Geometry: final body of the model. Coordinates: model frame, mm. Face numbers are marked on the shaded views. A direction names the side the tool comes from. Give positions to 0.01 mm unless a question says otherwise; leave off trailing zeros. Write each loop counter-clockwise with the first axis right and the second up, starting at its lowest first coordinate (ties: lowest second). Pieces come first, ordered by that corner, then holes.
Q1. Section D-D (y = 5.5). Return the cut outline in (x, z), plus the area to 3 significant figures.
Q2. Section B-B (x = 5). Return the cut outline in (y, z).
Q3. Reachability of the marked faces 4, 5 and 6 from +Z, -Z, +X, -X, +Y, -Y: full face, straight path, thin tool, end or side. Return the list, or none.
Q4. Pin query (flat end, axial travel): pin 1 Ø0.5 at (x, y) = (57.5, 1.5) entering from -Z; pin 2 Ø6 at (x, z) = (33.5, -56) entering from +Y; pin 3 Ø1 at (x, y) = (7.5, 2) entering from -Z. Return the tip coordinate at first contact, or that it passes through.
Q5. Line query: line 1 (Z direction, x = 24, y = 12.5); line 2 (X direction, y = 15, z = -29); line 3 (Z direction, x = 32, y = 11). Output: solid intervals per line, ascending.
Q6. Mould query, pull axis X, two halves, no side actions, for the marked faces 1, 2 and 3. Classes: +X half, -X half, draft (parallel to the pull), parting line (faces both ways), or undercut.
Q7. Section A-A (y = 12.25). Return the cut outline in (x, z).
Q8. Section C-C (z = -53.5). Return the cut outline in (x, y).
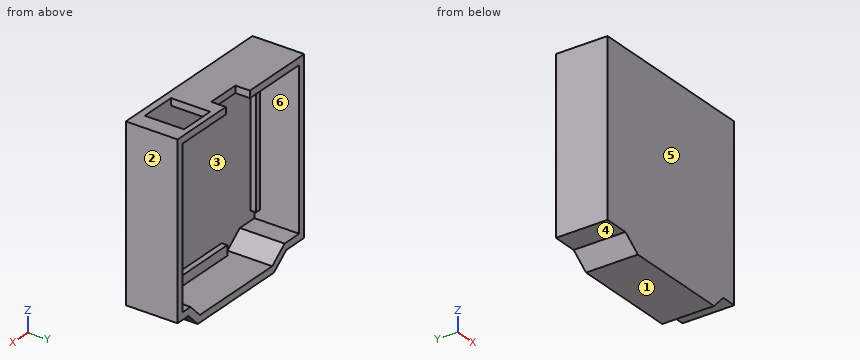
from build123d import *

# Parameters (mm, degrees)
BOSS_EXTRUDE1_DEPTH = 16
SHELL1_T            = 2.5
SKETCH2_W           = 13
SKETCH2_H           = 14
SKETCH2_W_2         = 12
SKETCH2_H_2         = 5.195244662
CUT_EXTRUDE1_DEPTH  = 4
SKETCH3_W           = 2
SKETCH3_H           = 50
SKETCH3_W_2         = 1.814522713
BOSS_EXTRUDE2_DEPTH = 2
SKETCH4_W           = 31.017616101
SKETCH4_H           = 3.530460369
BOSS_EXTRUDE3_DEPTH = 2


with BuildPart() as part:
    # Sketch1 → Boss-Extrude1 (new body)
    with BuildSketch(Plane(origin=(0, 0, 0), x_dir=(1, 0, 0), z_dir=(0, 1, 0))):
        Polygon((0, 0), (0, 56), (7.260584432, 56), (13.399361706, 60.750217247), (49.399361706, 60.750217247), (54, 56), (58, 56), (58, 0), align=None)
    extrude(amount=BOSS_EXTRUDE1_DEPTH)

    # Shell1
    shell1_openings = [part.faces().sort_by_distance(p)[0] for p in [
        (29.113999919, 16, -29.727085855),
    ]]
    offset(amount=SHELL1_T, openings=shell1_openings, kind=Kind.INTERSECTION)

    # Sketch2 → Cut-Extrude1 (cut)
    with BuildSketch(Plane(origin=(0, 0, 0), x_dir=(-1, 0, 0), z_dir=(0, 0, -1))):
        with Locations((-48, 7)):
            Rectangle(SKETCH2_W, SKETCH2_H)
        with Locations((-30.5, 13.402377669)):
            Rectangle(SKETCH2_W_2, SKETCH2_H_2)
    extrude(amount=-CUT_EXTRUDE1_DEPTH, mode=Mode.SUBTRACT)

    # Sketch3 → Boss-Extrude2 (add)
    with BuildSketch(Plane(origin=(0, 0, 0), x_dir=(1, 0, 0), z_dir=(0, 1, 0))):
        with Locations((1, 27.58353092)):
            Rectangle(SKETCH3_W, SKETCH3_H)
        with Locations((56.968981121, 27.58353092)):
            Rectangle(SKETCH3_W_2, SKETCH3_H)
    extrude(amount=BOSS_EXTRUDE2_DEPTH)

    # Sketch4 → Boss-Extrude3 (add)
    with BuildSketch(Plane(origin=(0, 0, 0), x_dir=(1, 0, 0), z_dir=(0, 1, 0))):
        with Locations((31.80262956, 58.741489624)):
            Rectangle(SKETCH4_W, SKETCH4_H)
    extrude(amount=BOSS_EXTRUDE3_DEPTH)


solid = part.part
Computed:
1. outline: (-2.5, -58.5) - (6.41, -58.5) - (12.55, -63.25) - (50.46, -63.25) - (55.06, -58.5) - (60.5, -58.5) - (60.5, 2.5) - (54.5, 2.5) - (54.5, 0) - (58, 0) - (58, -56) - (54, -56) - (49.4, -60.75) - (13.4, -60.75) - (7.26, -56) - (0, -56) - (0, 0) - (41.5, 0) - (41.5, 2.5) - (-2.5, 2.5) - close
1. area: 572 mm2
2. outline: (-2.5, -58.5) - (16, -58.5) - (16, -56) - (0, -56) - (0, 0) - (16, 0) - (16, 2.5) - (-2.5, 2.5) - close
3. face 4: -Z, -X, +Y, -Y
3. face 5: +Z, -Z, +X, -X, -Y
3. face 6: +Y
4. pin 1: stops at z = -58.5
4. pin 2: stops at y = 2
4. pin 3: stops at z = -59.73
5. line 1: z = -63.25 to -60.75, 0 to 2.5
5. line 2: x = -2.5 to 0, 58 to 60.5
5. line 3: z = -63.25 to -60.75
6. face 1: draft
6. face 2: +X half
6. face 3: undercut
7. outline: (-2.5, -58.5) - (6.41, -58.5) - (12.55, -63.25) - (50.46, -63.25) - (55.06, -58.5) - (60.5, -58.5) - (60.5, 2.5) - (54.5, 2.5) - (54.5, 0) - (58, 0) - (58, -56) - (54, -56) - (49.4, -60.75) - (13.4, -60.75) - (7.26, -56) - (0, -56) - (0, 0) - (24.5, 0) - (24.5, 2.5) - (-2.5, 2.5) - close; (36.5, 0) - (41.5, 0) - (41.5, 2.5) - (36.5, 2.5) - close
8. outline: (-2.5, -2.5) - (60.5, -2.5) - (60.5, 16) - (58, 16) - (58, 0) - (0, 0) - (0, 16) - (-2.5, 16) - close
